CAD build for the part. Positions are in the model's coordinates, mm. A direction names the side the tool comes from. Round coordinates to 2 decimals unless told otherwise and drop trailing zeros. Order: outer loops, then holes, each group sorted by start corner. A loop starts at its lowest first (then second) coordinate and runs counter-clockwise, first axis right, second up. Notation, with made-up numbers: M -1,26 L 29,26 A26 cw 29,49 Z; hole C -36.5,-16.5 d3. An arc over 180 degrees is marked long. Answer as a JSON object with one key per item and string values. Group by question number.
```python
from build123d import *

# Parameters (mm, degrees)
SKETCH2_R          = 1.6256
CUT_EXTRUDE1_DEPTH = 3.556
CIRPATTERN1_COUNT  = 4
CUT_EXTRUDE2_DEPTH = 3.556


with BuildPart() as part:
    # Sketch1 → Revolve1 (revolve)
    with BuildSketch(Plane.XY):
        Polygon((-15.1384, 4.99999), (-5.1384, 4.99999), (-5.1384, 11), (-1.5824, 11), (-1.5824, 5.08), (0, 5.08), (0, 4), (-15.1384, 4), align=None)
    revolve(axis=Axis((0, 0, 0), (-1, 0, 0)))

    # Sketch2 → Cut-Extrude1 (cut)
    with BuildSketch(Plane(origin=(-1.5824, 0, 0), x_dir=(0, 0, -1), z_dir=(1, 0, 0))):
        with Locations((0, 7.97105)):
            Circle(SKETCH2_R)
    cut_extrude1 = extrude(amount=-CUT_EXTRUDE1_DEPTH, mode=Mode.SUBTRACT)

    # CirPattern1: Cut-Extrude1 ×4 about axis
    cirpattern1_axis = Axis((0, 0, 0), (1, 0, 0))
    for i in range(1, CIRPATTERN1_COUNT):
        add(cut_extrude1.rotate(cirpattern1_axis, i * 360 / CIRPATTERN1_COUNT), mode=Mode.SUBTRACT)

    # Sketch3 → Cut-Extrude2 (cut)
    with BuildSketch(Plane(origin=(-1.5824, 0, 0), x_dir=(0, 0, -1), z_dir=(1, 0, 0))):
        with BuildLine():
            Line((-4.215969639, 10.16), (4.215969639, 10.16))
            ThreePointArc((4.215969639, 10.16), (0, 11), (-4.215969639, 10.16))
        make_face()
    extrude(amount=-CUT_EXTRUDE2_DEPTH, mode=Mode.SUBTRACT)


solid = part.part
```
Item 1: Cut at A-A, the plane z = 0. Give the cut face in (x, y), and give its area (3 significant figures).
Item 2: Drill centre lines: line 1 (Z direction, x = -4.35, y = 0); line 2 (X direction, y = 6, z = 3.75); line 3 (Y direction, x = -3.25, z = 1). Where is each one in solid material? Low to high. Write a range as [from, to].
Item 3: Flat gauge pins, fed straight in: pin 1 Ø3.5 at (y, z) = (-7.97, 0) entering from +X; pin 2 Ø1 at (y, z) = (6, -5.5) entering from -X; pin 3 Ø2 at (x, z) = (-10.5, -5) entering from -Y. Where does each tip first touch, or does it go through?
Item 4: 3-axis set-ups, long thin cutter, end or side, ignore diameter. For faces 1 (the face through (-3.336, -0.212, 9.583)), 2 (the face through (-5.138, -5, 2)), 3 (the face through (-0.78, -0.661, -5.037)): which of +Z, -Z, +X, -X, +Y, -Y reach the whole face in a straight line?
Item 5: Two-plate mould, pull along Z, no slides. Class faces 4 (the face through (-3, -11, 0)), 5 (the face through (-7.675, -0.867, 3.905)), 6 (the face through (-1.582, -5.3, -0.2)): +Z half, -Z half, draft (parallel to the pull), parting line (faces both ways), or undercut.
Item 6: Cut at C-C, the plane x = -8. Give the cut face in (y, z), and give its area (3 significant figures).
Item 7: Cut at B-B, the plane y = 0. Give the cut face in (x, z).
Item 8: Cut at D-D, the plane z = 8.75. Give the cut face in (x, y).
Response values:
{
 "1": {"outline": "M -15.14,-5 L -5.14,-5 L -5.14,-6.35 L -1.58,-6.35 L -1.58,-5.08 L 0,-5.08 L 0,-4 L -15.14,-4 Z; M -15.14,4 L 0,4 L 0,5.08 L -1.58,5.08 L -1.58,6.35 L -5.14,6.35 L -5.14,5 L -15.14,5 Z; M -5.14,-11 L -1.58,-11 L -1.58,-9.6 L -5.14,-9.6 Z; M -5.14,9.6 L -1.58,9.6 L -1.58,10.16 L -5.14,10.16 Z", "area": "47.1 mm^2"},
 "2": {"line 1": "[-11, -9.6], [-6.35, -4], [4, 6.35], [9.6, 11]", "line 2": "[-5.14, -1.58]", "line 3": "[-10.95, -9.25], [-6.69, -3.87], [3.87, 6.69], [9.25, 10.16]"},
 "3": {"pin 1": "x = -1.58", "pin 2": "x = -5.14", "pin 3": "y = -3"},
 "4": {"face 1": "+X, -X", "face 2": "-X", "face 3": "+X"},
 "5": {"face 4": "parting line", "face 5": "undercut", "face 6": "draft"},
 "6": {"outline": "C 0,0 d10; hole C 0,0 d8", "area": "28.3 mm^2"},
 "7": {"outline": "M -15.14,-5 L -5.14,-5 L -5.14,-6.35 L -1.58,-6.35 L -1.58,-5.08 L 0,-5.08 L 0,-4 L -15.14,-4 Z; M -15.14,4 L 0,4 L 0,5.08 L -1.58,5.08 L -1.58,6.35 L -5.14,6.35 L -5.14,5 L -15.14,5 Z; M -5.14,-11 L -1.58,-11 L -1.58,-9.6 L -5.14,-9.6 Z; M -5.14,9.6 L -1.58,9.6 L -1.58,11 L -5.14,11 Z"},
 "8": {"outline": "M -5.14,-6.67 L -1.58,-6.67 L -1.58,-1.43 L -5.14,-1.43 Z; M -5.14,1.43 L -1.58,1.43 L -1.58,6.67 L -5.14,6.67 Z"}
}
